from build123d import *

# Parameters (mm, degrees)
F0_W     = 110
F0_H     = 200
F1_DEPTH = 10
F2_R     = 10
F3_DEPTH = 40
F4_W     = 110
F4_H     = 200
F5_DEPTH = 10
F6_R     = 10
F7_DEPTH = 19
F8_R     = 10
F9_DEPTH = 19


with BuildPart() as f1:
    # F0 (on Front) → F1 (new body)
    with BuildSketch(Plane.XZ):
        Rectangle(F0_W, F0_H)
    extrude(amount=F1_DEPTH)

    # F2 (on face) → F3 (join)
    with BuildSketch(Plane.XZ.offset(10)):
        with Locations((55, 0)):
            Circle(F2_R)
    extrude(amount=F3_DEPTH)

    # F4 (on face) → F5 (join)
    with BuildSketch(Plane.XZ.offset(50)):
        Rectangle(F4_W, F4_H)
    extrude(amount=F5_DEPTH)

    # F6 (on face) → F7 (join)
    with BuildSketch(Plane.XZ.offset(10)):
        with Locations((-55, 0)):
            Circle(F6_R)
    extrude(amount=F7_DEPTH)

    # F8 (on face) → F9 (join)
    with BuildSketch(Plane(origin=(0, -50, 0), x_dir=(-1, 0, 0), z_dir=(0, 1, 0))):
        with Locations((55, 0)):
            Circle(F8_R)
    extrude(amount=F9_DEPTH)


solid = f1.part
Build history of the part. All positions in model axes, mm. A direction names the side the tool comes from. Give positions to 0.01 mm unless a question says otherwise; leave off trailing zeros. Order: outer loops, then holes, each group sorted by start corner. A loop starts at its lowest first (then second) coordinate and runs counter-clockwise, first axis right, second up. Notation, with made-up numbers: M 57,-1 L 86,-1 A16 cw 86,16 Z; hole C 56.25,82 d6. An arc over 180 degrees is marked long. Use one line per item in the form item = value.
Q1. Pull direction Y, two halves, no side cores. Call faces 5 (the cylindrical face through (45, -30, 0)), 6 (the flat face through (-1, 0, 1)), 7 (the flat face through (-55, -31, 0)), 8 (the flat face through (-59, -50, 0)): released by +Y, released by -Y, zero draft, split by the parting line, or undercut.
Conclusion:
face_5 = undercut
face_6 = released by +Y
face_7 = undercut
face_8 = released by -Y
Q2. Which spindle directions (+Z, -Z, +X, -X, +Y, -Y) get a long thin tool onto all of the face, cutting with end or side? Do faces 1 (the flat face through (-55, -29, 0)), 2 (the cylindrical face through (-45, -41, 0)), 3 (the flat face through (59, -10, 0)), 4 (the flat face through (59, -50, 0)). Say none if no direction does.
Conclusion:
face_1 = +Z, -Z, -X
face_2 = none
face_3 = +Z, -Z, +X, +Y
face_4 = +Z, -Z, +X, -Y
Q3. Slice it at D-D, the plane y = -22. Write the cut outline in (x, z), and give its area (3 significant figures).
Conclusion:
outline = C -55,0 d20; C 55,0 d20
area = 628 mm2
Q4. Slice it at B-B, the plane z = 76. Write the cut outline in (x, y), and give its area (3 significant figures).
Conclusion:
outline = M -55,-60 L 55,-60 L 55,-50 L -55,-50 Z; M -55,-10 L 55,-10 L 55,0 L -55,0 Z
area = 2,200 mm2
Q5. Slice it at C-C, the plane z = -6. Write the cut outline in (x, y).
Conclusion:
outline = M -63,-50 L -55,-50 L -55,-60 L 55,-60 L 55,-50 L 63,-50 L 63,-10 L 55,-10 L 55,0 L -55,0 L -55,-10 L -63,-10 L -63,-29 L -47,-29 L -47,-10 L 47,-10 L 47,-50 L -47,-50 L -47,-31 L -63,-31 Z
Q6. Slice it at A-A, the plane x = -8.5. Write the cut outline in (y, z), and give its area (3 significant figures).
Conclusion:
outline = M -60,-100 L -50,-100 L -50,100 L -60,100 Z; M -10,-100 L 0,-100 L 0,100 L -10,100 Z
area = 4,000 mm2
Q7. Pin check, flat tips, straight feed: P1, Ø12, axis at x = -17.5, z = 20, coming from the +Y side; P2, Ø5, axis at y = -53.5, z = -2, coming from the +X side; P3, Ø8, axis at x = 61, z = -4, coming from the -Y side; P4, Ø5, axis at x = -61, z = 1.5, coming from the +Y side. Stop position of each tip, or through.
Conclusion:
P1 = 0
P2 = 55
P3 = -50
P4 = -10
Q8. Wall check: probe 1 along Y at (x, z) = (-20, -71); probe 2 along X at (y, z) = (-5, -78); probe 3 along Z at (x, y) = (-51, -46). Give the ranges that are in metal, low to high.
Conclusion:
probe_1 = -60 to -50, -10 to 0
probe_2 = -55 to 55
probe_3 = -9.17 to 9.17
